The model under review builds one solid part; all positions refer to its coordinate system, in mm. Give positions to 0.01 mm unless a question says otherwise; leave off trailing zeros. Order: outer loops, then holes, each group sorted by start corner. A loop starts at its lowest first (then second) coordinate and runs counter-clockwise, first axis right, second up.
```python
from build123d import *

# Parameters (mm, degrees)
F1_DEPTH = 50
F2_T     = -4
F3_R     = 5
F4_D     = 22


with BuildPart() as f1:
    # F0 (on Right) → F1 (new body)
    with BuildSketch(Plane.YZ):
        Polygon((-52.4746724886, 274.1746123904), (-52.4746724886, -325.8253876096), (47.5253275114, -375.8253876096), (47.5253275114, 324.1746123904), align=None)
    extrude(amount=F1_DEPTH)

    # F2
    f2_openings = [f1.faces().sort_by_distance(p)[0] for p in [
        (25, -2.474672, -350.825388),
    ]]
    offset(amount=F2_T, openings=f2_openings)

    # F3
    f3_edges = [f1.edges().sort_by_distance(p)[0] for p in [
        (50, -52.474672, -25.825388),
        (50, 47.525328, -25.825388),
        (0, 47.525328, -25.825388),
        (0, -52.474672, -25.825388),
        (4, -48.474672, -28.061456),
        (4, 43.525328, -28.061456),
        (46, 43.525328, -28.061456),
        (46, -48.474672, -28.061456),
    ]]
    fillet(f3_edges, radius=F3_R)

    # F4 (through all)
    with Locations(Plane(origin=(0, 0, 0), x_dir=(0, 1, 0), z_dir=(-1, 0, 0))):
        with Locations((0, 125.8253876096)):
            Hole(F4_D / 2)


solid = f1.part
```
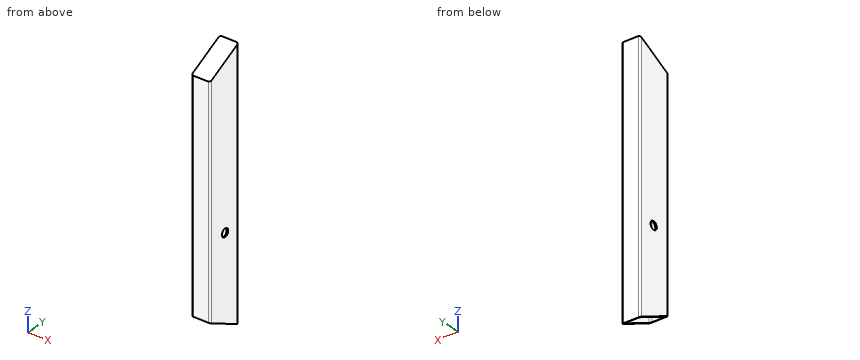
Item 1: Take a section at C-C (y = 0). Give the boundary of the cut face in (x, z), and give its area (3 significant figures).
Values found:
outline: (0, -352.06) - (4, -352.06) - (4, -136.83) - (0, -136.83) - close; (0, -114.83) - (4, -114.83) - (4, 295.94) - (46, 295.94) - (46, -114.83) - (50, -114.83) - (50, 300.41) - (0, 300.41) - close; (46, -352.06) - (50, -352.06) - (50, -136.83) - (46, -136.83) - close
area: 5,230 mm2
Item 2: Clearance check with flat-ended pins moving along their axes: pin 1 Ø8 at (x, y) = (9, -26.5) entering from +Z; pin 2 Ø5 at (x, y) = (34.5, 4) entering from +Z; pin 3 Ø20 at (y, z) = (0, -125.83) entering from -X. State where each tip first meets the part, or that it passes through.
Values found:
pin 1: stops at z = 289.16
pin 2: stops at z = 303.66
pin 3: passes through
Item 3: Take a section at A-A (z = -310.5). Give the boundary of the cut face in (x, y), and give its area (3 significant figures).
Values found:
outline: (0, -47.47) arc R5 ccw to (5, -52.47) - (45, -52.47) arc R5 ccw to (50, -47.47) - (50, 42.53) arc R5 ccw to (45, 47.53) - (5, 47.53) arc R5 ccw to (0, 42.53) - close; hole (4, -43.47) arc R5 ccw to (9, -48.47) - (41, -48.47) arc R5 ccw to (46, -43.47) - (46, 38.53) arc R5 ccw to (41, 43.53) - (9, 43.53) arc R5 ccw to (4, 38.53) - close
area: 1,140 mm2
Item 4: Take a section at B-B (x = 25). Give the boundary of the cut face in (y, z).
Values found:
outline: (-52.47, -325.83) - (-48.47, -327.83) - (-48.47, 271.7) - (43.53, 317.7) - (43.53, -373.83) - (47.53, -375.83) - (47.53, 324.17) - (-52.47, 274.17) - close
Item 5: For line 1 (X direction, y = -36, z = -288); line 2 (Y direction, x = 15.5, z = 262.5); line 3 (Y direction, x = 42, z = 223.5), list the stretches that pass through material, from the lowest coordinate up.
Values found:
line 1: x = 0 to 4, 46 to 50
line 2: y = -52.47 to -48.47, 43.53 to 47.53
line 3: y = -52.47 to -48.37, 43.42 to 47.53
